Autodesk Inventor part; units mm, degrees
ref_plane "YZ Plane" through (0, 0, 0) normal (1, 0, 0) x (0, 1, 0)
ref_plane "XZ Plane" through (0, 0, 0) normal (0, 1, 0) x (-1, 0, 0)
ref_plane "XY Plane" through (0, 0, 0) normal (0, 0, 1) x (1, 0, 0)
sketch "草图1" plane through (0, 0, 0) normal (1, 0, 0) x (0, 1, 0)
  circle A0 centre (0, 0) radius 12.5
  dimension "d0" = 25
extrude "拉伸1" add sketch "草图1" along normal blind 75
sketch "草图2" plane through (0, 0, 0) normal (0, 1, 0) x (-1, 0, 0)
  circle A0 centre (-37.5, 0) radius 12.5
  line L0 (0, 12.5) -> (-75, 12.5)
  line L1 (0, -12.5) -> (-75, -12.5)
  point P0 (0, 0)
  point P1 (-37.5, -12.5)
extrude "拉伸2" add sketch "草图2" along normal mid plane 75
properties part number "第一次上机-示例建模"
The model under review builds one solid part; all positions refer to its coordinate system, in mm. A direction names the side the tool comes from. Give positions to 0.01 mm unless a question says otherwise; leave off trailing zeros. Loops run counter-clockwise (first coordinate to the right, second up) from the corner with the lowest first, then second, coordinate; pieces in that order, holes last. Notation, with made-up numbers: (-27, 44) -> (20, 44) arc R20 cw to (20, 64) -> close; hole circle Ø5 at (50, -11). An arc over 180 degrees is marked (long way). Write each question's results on one line, items separated by ' | '.
1) Tool access review of faces 1 (the face through (49.988, 22.654, -0.55)), 2 (the face through (14.321, -12.488, -0.55)), 3 (the face through (49.988, -22.654, 0.55)), 4 (the face through (60.154, -12.488, -0.55)): name each direction out of +Z, -Z, +X, -X, +Y, -Y from which nothing blocks a thin tool from reaching the whole face with its end or side.
Conclusion:
face 1: +Y | face 2: -X | face 3: -Y | face 4: +X
2) For line 1 along Y through (x, z) = (17.5, -0.25); line 2 along X through (y, z) = (-26, 0.75); line 3 along Z through (x, y) = (34, 31.5), list the stretches that pass through material, from the lowest coordinate up. Write a range as from..to.
Conclusion:
line 1: y = -12.5..12.5 | line 2: x = 25.02..49.98 | line 3: z = -12..12
3) Take a section at C-C, the plane x = 17. Give the boundary of the cut face in (y, z), plus the area to 3 significant figures.
Conclusion:
outline: circle Ø25 at (0, 0) | area: 491 mm^2
4) Take a section at D-D, the plane z = -4.25. Give the boundary of the cut face in (x, y), plus the area to 3 significant figures.
Conclusion:
outline: (0, -11.76) -> (25.74, -11.76) -> (25.74, -37.5) -> (49.26, -37.5) -> (49.26, -11.76) -> (75, -11.76) -> (75, 11.76) -> (49.26, 11.76) -> (49.26, 37.5) -> (25.74, 37.5) -> (25.74, 11.76) -> (0, 11.76) -> close | area: 2,970 mm^2
5) Insertion check: pin 1 Ø4 at (y, z) = (-15, -8) entering from +X; pin 2 Ø1 at (y, z) = (21, -3) entering from +X; pin 3 Ø10 at (x, z) = (53, -8.5) entering from +Y. Each pin has a flat end and moves straight along its axis. Give the tip position at first contact, or say it passes through.
Conclusion:
pin 1: stops at x = 48.47 | pin 2: stops at x = 49.75 | pin 3: stops at y = 12
6) Take a section at B-B, the plane y = 11.5. Give the boundary of the cut face in (x, z), plus the area to 3 significant figures.
Conclusion:
outline: (0, -4.9) -> (26, -4.9) arc R12.5 ccw to (49, -4.9) -> (75, -4.9) -> (75, 4.9) -> (49, 4.9) arc R12.5 ccw to (26, 4.9) -> (0, 4.9) -> close | area: 987 mm^2
7) Take a section at A-A, the plane z = 1.25. Give the boundary of the cut face in (x, y), plus the area to 3 significant figures.
Conclusion:
outline: (0, -12.44) -> (25.06, -12.44) -> (25.06, -37.5) -> (49.94, -37.5) -> (49.94, -12.44) -> (75, -12.44) -> (75, 12.44) -> (49.94, 12.44) -> (49.94, 37.5) -> (25.06, 37.5) -> (25.06, 12.44) -> (0, 12.44) -> close | area: 3,110 mm^2
